```python
from build123d import *

# Parameters (mm, degrees)
SKETCH_W     = 12
SKETCH_H     = 12
PAD_DEPTH    = 5
SKETCH001_R  = 3.2
POCKET_DEPTH = 10.001


with BuildPart() as body001:
    # Sketch002 → Revolution (revolve)
    with BuildSketch(Plane.XZ):
        Polygon((-6, 0), (-6, 1.9), (-5, 1.9), (-3.7, 3.2), (6, 3.2), (6, 0), align=None)
    revolve(axis=Axis((0, 0, 0), (1, 0, 0)))


with BuildPart() as cut:
    # Sketch → Pad (new body, symmetric)
    with BuildSketch(Plane.XY):
        Rectangle(SKETCH_W, SKETCH_H)
    extrude(amount=PAD_DEPTH, both=True)

    # Sketch001 (on Face6 of Pad) → Pocket (cut, through all)
    with BuildSketch(Plane.XY.offset(5)):
        with Locations((1, 0)):
            Circle(SKETCH001_R)
    extrude(amount=-POCKET_DEPTH, mode=Mode.SUBTRACT)

    # Cut: cut Body001
    add(body001.part, mode=Mode.SUBTRACT)


solid = cut.part
```
Check sheet for the modelled part. Datum: model origin and axes. Units: mm. A direction names the side the tool comes from. Give positions to 0.01 mm unless a question says otherwise; leave off trailing zeros. Order: outer loops, then holes, each group sorted by start corner. A loop starts at its lowest first (then second) coordinate and runs counter-clockwise, first axis right, second up. Notation, with made-up numbers: (22.25, -8.75) -> (43.25, -8.75) arc R28 cw to (43.25, 15.25) -> close; hole circle Ø5 at (-2, -16.75). An arc over 180 degrees is marked (long way). Use CSV: the item, a comma, the result in double quotes. Start each with the question number.
1) Sectioned sample at B-B, the plane x = -4. Record the boundary of the cut face in (y, z), plus the area to 3 significant figures.
2) Set-up check for faces 1 (the face through (4.646, -0.961, 3.052)), 2 (the face through (0.583, 3.173, -3.576)): record each of +Z, -Z, +X, -X, +Y, -Y from which the full face is reachable in a straight line by a thin tool's end or side.
3) Sectioned sample at D-D, the plane y = -1.5. Give the number of separate pieces and of enclosed holes in the cut face, plus the area to 3 significant figures.
4) Sectioned sample at A-A, the plane y = 0. Record the boundary of the cut face in (x, z), plus the area to 4 significant figures.
5) Go/stop test with flat-tipped pins: P1, Ø1, axis at y = 1.5, z = 2.5, coming from the +X side; P2, Ø6, axis at y = 0, z = 0, coming from the +X side. Record where each tip stops, or that it passes through.
6) Sectioned sample at C-C, the plane x = 0.25. Record the boundary of the cut face in (y, z), plus the area to 3 significant figures.
7) Material ranges on line 1 (Y direction, x = 1, z = 2.45); line 2 (Z direction, x = -5.45, y = 0); line 3 (Y direction, x = -5.7, z = 0), recorded low to high. Write a range as from..to.
8) Mould release check, pull along Y, two halves, no side actions. Record for faces 3 (the face through (-6, -0.1, 2.3)), 4 (the face through (0, -6, 0)), 5 (the face through (0, 6, 0)), 6 (the face through (4.052, 0.961, 3.646)): released by +Y, released by -Y, zero draft, split by the parting line, or undercut.
Recorded:
1,outline,"(-6, -5) -> (6, -5) -> (6, 5) -> (-6, 5) -> close; hole circle Ø5.8 at (0, 0)"
1,area,"93.6 mm2"
2,face 1,"+X"
2,face 2,"+Z, -Z"
3,separate pieces,"4"
3,enclosed holes,"0"
3,area,"32.9 mm2"
4,outline,"(-6, -5) -> (-2.2, -5) -> (-2.2, -3.2) -> (-3.7, -3.2) -> (-5, -1.9) -> (-6, -1.9) -> close; (-6, 1.9) -> (-5, 1.9) -> (-3.7, 3.2) -> (-2.2, 3.2) -> (-2.2, 5) -> (-6, 5) -> close; (4.2, -5) -> (6, -5) -> (6, -3.2) -> (4.2, -3.2) -> close; (4.2, 3.2) -> (6, 3.2) -> (6, 5) -> (4.2, 5) -> close"
4,area,"24.45 mm2"
5,P1,"x = 6"
5,P2,"x = -3.9"
6,outline,"(-6, -5) -> (-3.11, -5) -> (-3.11, -0.75) arc R3.2 cw to (-3.11, 0.75) -> (-3.11, 5) -> (-6, 5) -> close; (3.11, -5) -> (6, -5) -> (6, 5) -> (3.11, 5) -> (3.11, 0.75) arc R3.2 cw to (3.11, -0.75) -> close"
6,area,"57.6 mm2"
7,line 1,"-6..-3.2, 3.2..6"
7,line 2,"-5..-1.9, 1.9..5"
7,line 3,"-6..-1.9, 1.9..6"
8,face 3,"zero draft"
8,face 4,"released by -Y"
8,face 5,"released by +Y"
8,face 6,"undercut"
